Autodesk Inventor part; units mm, degrees
ref_plane "Work Plane1" through (-20, 0, 0) normal (1, 0, 0) x (0, 0, -1)
ref_plane "YZ Plane" through (0, 0, 0) normal (1, 0, 0) x (0, 1, 0)
ref_plane "XZ Plane" through (0, 0, 0) normal (0, 1, 0) x (-1, 0, 0)
sketch "Sketch1" plane through (0, 0, 0) normal (1, 0, 0) x (0, 1, 0)
  line L0 (0, 0) -> (0, -300)
  line L1 (0, 0) -> (103.9616, -241.9966)
  line L2 (431.1742, -241.9966) -> (207.8735, -323.7914)
  arc A0 (0, -300) -> (207.8735, -323.7914) centre (114.5573, -219.1004) ccw
  line L3 (103.9616, -241.9966) -> (492.1494, -162.4552)
  line L4 (492.1494, -162.4552) -> (431.1742, -241.9966)
  dimension "d5" = 300
extrude "Extrusion1" add sketch "Sketch1" against normal blind 500
ref_plane "Work Plane1" through (-20, 0, 0) normal (1, 0, 0) x (0, 0, -1)
sketch "Sketch2" plane through (-20, 0, 0) normal (1, 0, 0) x (0, 0, -1)
  line L0 (292.8468, 11.7995) -> (-65.8674, 11.7995)
  line L1 (170.4104, 471.7728) -> (314.1993, 195.7664)
  arc A0 (290.3714, 11.7995) -> (314.1993, 195.7664) centre (219.1004, 114.5573) ccw
  arc A1 (300, 0) -> (323.7914, 207.8735) centre (219.1004, 114.5573) ccw
  line L2 (-61.2921, 11.7995) -> (-54.1186, 588.7001)
  line L3 (-54.1186, 588.7001) -> (170.4104, 471.7728)
  point P0 (0, 0)
  dimension "d9" = 250.1097
extrude "Extrusion2" cut sketch "Sketch2" against normal blind 460
sketch "Sketch3" plane through (0, 0, 0) normal (1, 0, 0) x (0, 0, -1)
  line L0 (269.1004, 100) -> (309.1004, 100)
  line L1 (309.1004, 100) -> (309.1004, 60)
  line L2 (309.1004, 60) -> (269.1004, 60)
  line L3 (269.1004, 60) -> (269.1004, 100)
  line L4 (0, 0) -> (300, 0)
  arc A0 (300, 0) -> (323.7914, 207.8735) centre (219.1004, 114.5573) ccw
  dimension "d12" = 40
  dimension "d13" = 40
  dimension "d14" = 60
  dimension "d15" = 90
extrude "Extrusion3" add sketch "Sketch3" along normal blind 50
sketch "Sketch4" plane through (50, 0, 0) normal (1, 0, 0) x (0, 0, -1)
  line L0 (309.1004, 100) -> (269.1004, 100)
  line L1 (269.1004, 100) -> (269.1004, 60)
  line L2 (269.1004, 60) -> (309.1004, 60)
  line L3 (309.1004, 60) -> (309.1004, 100)
  line L4 (259.1004, 110) -> (319.1004, 110)
  line L5 (319.1004, 110) -> (319.1004, 50)
  line L6 (319.1004, 50) -> (259.1004, 50)
  line L7 (259.1004, 50) -> (259.1004, 110)
  point P0 (0, 0)
  dimension "d18" = 60
  dimension "d19" = 60
  dimension "d20" = 10
  dimension "d21" = 10
extrude "Extrusion4" add sketch "Sketch4" along normal blind 10 contours L3 L2 L1 L0 | L4 L5 L6 L7
sketch "Sketch5" plane through (-500, 0, 0) normal (-1, 0, 0) x (0, 0, 1)
  line L0 (-309.1004, 100) -> (-269.1004, 100)
  line L1 (-269.1004, 100) -> (-269.1004, 60)
  line L2 (-269.1004, 60) -> (-309.1004, 60)
  line L3 (-309.1004, 60) -> (-309.1004, 100)
  arc A0 (-323.7914, 207.8735) -> (-300, 0) centre (-219.1004, 114.5573) ccw
  line L4 (-300, 0) -> (0, 0)
  dimension "d24" = 40
  dimension "d25" = 40
  dimension "d26" = 90
  dimension "d27" = 60
extrude "Extrusion5" add sketch "Sketch5" along normal blind 50
sketch "Sketch6" plane through (-550, 0, 0) normal (-1, 0, 0) x (0, 0, 1)
  point P0 (0, 0)
sketch "Sketch7" plane through (-550, 0, 0) normal (-1, 0, 0) x (0, 0, 1)
  point P0 (0, 0)
sketch "Sketch8" plane through (-550, 0, 0) normal (-1, 0, 0) x (0, 0, 1)
  line L0 (-269.1004, 100) -> (-309.1004, 100)
  line L1 (-309.1004, 100) -> (-309.1004, 60)
  line L2 (-309.1004, 60) -> (-269.1004, 60)
  line L3 (-269.1004, 60) -> (-269.1004, 100)
  line L4 (-319.1004, 110) -> (-259.1004, 110)
  line L5 (-259.1004, 110) -> (-259.1004, 50)
  line L6 (-259.1004, 50) -> (-319.1004, 50)
  line L7 (-319.1004, 50) -> (-319.1004, 110)
  point P0 (0, 0)
  dimension "d30" = 60
  dimension "d31" = 60
  dimension "d33" = 10
  dimension "d34" = 10
extrude "Extrusion6" add sketch "Sketch8" along normal blind 10 contours L3 L2 L1 L0 | L4 L5 L6 L7
properties part number "hoe me"
The listing builds one solid part. Answer for the finished solid, in the listing's coordinates (mm). A direction names the side the tool comes from. Coordinates: 2 decimals unless noted, no trailing zeros. Loops run counter-clockwise (first coordinate to the right, second up) from the corner with the lowest first, then second, coordinate; pieces in that order, holes last. Notation, with made-up numbers: (-33.75, 83.5) -> (-25.75, 83.5) arc R28 ccw to (-25.75, 112.5) -> close; hole circle Ø9 at (77.5, -33.75). An arc over 180 degrees is marked (long way). Use one line per item in the form item = value. Start each with the question number.
Item 1: The part is cut by section C-C on y = 185. Determine the outline of the cut face in (x, z), then the cut area to 3 significant figures.
Item 2: A tool of negligible diameter and unlimited length cuts with its end or side. For faces 1 (the face through (25, 80, -309.1)), 2 (the face through (-525, 100, -289)), 3 (the face through (50, 100.4, -288.7)), 4 (the face through (-247, 11.8, -161)), 5 (the face through (25, 60, -289)), from which of +Z, -Z, +X, -X, +Y, -Y can it reach the whole face along a straight path? Write none if from no direction.
Item 3: The part is cut by section A-A on x = -302. Determine the outline of the cut face in (y, z), then the cut area to 3 significant figures.
Item 4: The part is cut by section B-B on z = -189.5. Determine the outline of the cut face in (x, y), then the cut area to 3 significant figures.
Item 5: Consider L1, parallel to X at y = 91, z = -264; L2, parallel to X at y = 327.5, z = -196.5; L3, parallel to Y at x = -151, z = -43.5. Determine where each line is inside the solid, lowest interval first. Write a range as [from, to].
Item 6: The mould has two halves that part along X. Classify faces 6 (the face through (60, 80, -289)), 7 (the face through (-248.833, 9.383, -21.842)), 8 (the face through (-525, 80, -309.1)), 9 (the face through (-246.8, 335.7, -241.3)): released by +X, released by -X, zero draft, split by the parting line, or undercut.
Item 7: Flat-ended cylindrical pins translate along their axes: pin 1 Ø8 at (x, z) = (-105, -323) entering from -Y; pin 2 Ø20 at (x, y) = (-532.5, 76.5) entering from +Z; pin 3 Ø8 at (x, z) = (-260.5, -44.5) entering from +Y. Find the tip coordinate at first contact, or state that the pin passes through.
Item 8: The part is cut by section D-D on z = -38. Determine the outline of the cut face in (x, y).
Answer key:
q1.outline = (-500, -340.37) -> (0, -340.37) -> (0, -225.39) -> (-20, -225.39) -> (-20, -322.43) -> (-480, -322.43) -> (-480, -225.39) -> (-500, -225.39) -> close
q1.area = 12,900 mm2
q2.face_1 = -Z, +Y, -Y
q2.face_2 = +Z, -Z, +Y
q2.face_3 = none
q2.face_4 = +Z
q2.face_5 = +Z, -Z, -Y
q3.outline = (0, -300) arc R140.24 ccw to (207.87, -323.79) -> (431.17, -242) -> (492.15, -162.46) -> (473.98, -166.18) -> (471.77, -170.41) -> (195.77, -314.2) arc R125.05 cw to (11.8, -290.37) -> (11.8, -27.47) -> (0, 0) -> close
q3.area = 15,800 mm2
q4.outline = (-500, 0) -> (0, 0) -> (0, 81.41) -> (-20, 81.41) -> (-20, 11.8) -> (-480, 11.8) -> (-480, 81.41) -> (-500, 81.41) -> close; (-500, 360.16) -> (-480, 360.16) -> (-480, 435.13) -> (-20, 435.13) -> (-20, 360.16) -> (0, 360.16) -> (0, 471.42) -> (-500, 471.42) -> close
q4.area = 29,800 mm2
q5.L1 = [-560, -550], [-500, -480], [-20, 0], [50, 60]
q5.L2 = [-500, -480], [-20, 0]
q5.L3 = [0, 11.8]
q6.face_6 = released by +X
q6.face_7 = zero draft
q6.face_8 = undercut
q6.face_9 = undercut
q7.pin_1 = 16.13
q7.pin_2 = -269.1
q7.pin_3 = 11.8
q8.outline = (-500, 0) -> (0, 0) -> (0, 16.32) -> (-20, 16.32) -> (-20, 11.8) -> (-480, 11.8) -> (-480, 16.32) -> (-500, 16.32) -> close
